Check sheet for the modelled part. Datum: model origin and axes. Units: mm. A direction names the side the tool comes from. Round coordinates to 2 decimals unless told otherwise and drop trailing zeros. Loops run counter-clockwise (first coordinate to the right, second up) from the corner with the lowest first, then second, coordinate; pieces in that order, holes last. Notation, with made-up numbers: (-33, -39.5) - (-12, -39.5) arc R29 ccw to (-12, -7.5) - close; hole circle Ø7 at (10, -29.75). An arc over 180 degrees is marked (long way). Answer in a Markdown table with one row per item. Add a question column.
(1) Cross-section at B-B on z = 0. Enter the section's corners in (x, y), then the cut area to 3 significant figures.
(2) Thickness scan on line 1 along Z through (x, y) = (2.25, 0); line 2 along Z through (x, y) = (-4.25, 4); line 3 along Z through (x, y) = (3.5, 5). Record the ranges inside material, lowest first.
(3) Cross-section at C-C on x = -5. Enter the section's corners in (y, z).
(4) Mould release check, pull along Z, two halves, no side actions. Record for faces 1 (the cylindrical face through (2.46, -0.01, -8.75)), 2 (the flat face through (-8, 2.2, -2.2)), 3 (the cylindrical face through (2.465, 9.895, -0.825)): +Z half, -Z half, draft (parallel to the pull), parting line (faces both ways), or undercut.
(5) Cross-section at A-A on y = 0. Enter the section's corners in (x, z), then the cut area to 3 significant figures.
(6) Access from +Z, -Z, +X, -X, +Y, -Y to the whole of each face (thin tool, end or side, straight path). Record for faces 4 (the cylindrical face through (-3.51, 3.56, -1.62)), 5 (the cylindrical face through (2.465, -7.502, -6.457)), 6 (the cylindrical face through (2.465, -0.825, -9.895)), 7 (the cylindrical face through (2.46, 7.08, 5.14)).
(7) Gauge pin test, flat ends, axial feed: pin 1 (10 mm diameter, centred on y = 3, z = 7, fed in from -X); pin 2 (1.1 mm diameter, centred on x = -6, z = 0, fed in from -Y); pin 3 (3 mm diameter, centred on y = -6.5, z = 6.5, fed in from -X); pin 4 (3 mm diameter, centred on x = -3, z = 0, fed in from +Y). Record the tip position at first contact, or that the pin passes through.
(8) Cross-section at D-D on y = -4. Enter the section's corners in (x, z).
from build123d import *

# Parameters (mm, degrees)
BASPROSKE_W             = 5
BASPROSKE_H             = 11
TOOTHCUT_DEPTH          = 17.340134638
TEETHCUTS_COUNT         = 20
TEETHCUTS_ANGLE         = 342
HUBNEAONESKE_R          = 5
HUBNEARONE_DEPTH        = 10.0000508
BORSKE_R                = 3
BORE_DEPTH              = 15.0000508
BOSS_EXTRUDE1_START     = -10.000051
SKETCH2_R               = 3
BOSS_EXTRUDE1_DEPTH     = 15.0000508
SKETCH3_R               = 1.7
CUT_EXTRUDE1_DEPTH      = 10
SKETCH4_W               = 2
SKETCH4_H               = 20.201666504
CUT_EXTRUDE2_DEPTH      = 19.39087628
CUT_EXTRUDE2_DEPTH_BACK = 19.39087628
CUT_EXTRUDE3_DEPTH      = 31


with BuildPart() as part:
    # BasProSke → Base-Revolve (revolve)
    with BuildSketch(Plane(origin=(0, 0, 0), x_dir=(1, 0, 0), z_dir=(0, 1, 0)), mode=Mode.PRIVATE) as base_revolve_sk:
        with Locations((2.5, 5.5)):
            Rectangle(BASPROSKE_W, BASPROSKE_H)
    revolve(base_revolve_sk.sketch.rotate(Axis((-10, 0, 0), (1, 0, 0)), 180), axis=Axis((-10, 0, 0), (1, 0, 0)))

    # TooCutSke → ToothCut (cut, through all)
    with BuildSketch(Plane(origin=(0, 0, 0), x_dir=(0, 0, -1), z_dir=(1, 0, 0))):
        with BuildLine():
            ThreePointArc((0.589353609, 8.729127295), (0, 8.749), (-0.589353609, 8.729127295))
            ThreePointArc((-0.589353609, 8.729127295), (-0.82475631, 9.893403384), (-1.391689312, 10.937213814))
            ThreePointArc((-1.391689312, 10.937213814), (0, 11.0254), (1.391689312, 10.937213814))
            ThreePointArc((1.391689312, 10.937213814), (0.82475631, 9.893403384), (0.589353609, 8.729127295))
        make_face()
    toothcut = extrude(amount=TOOTHCUT_DEPTH, mode=Mode.SUBTRACT)

    # TeethCuts: ToothCut ×20 about axis
    teethcuts_axis = Axis((-10, 0, 0), (1, 0, 0))
    for i in range(1, TEETHCUTS_COUNT):
        add(toothcut.rotate(teethcuts_axis, i * TEETHCUTS_ANGLE / (TEETHCUTS_COUNT - 1)), mode=Mode.SUBTRACT)

    # HubNeaOneSke → HubNearOne (add)
    with BuildSketch(Plane.ZY):
        with Locations(Location((0, 0, 0), (0, 0, 180))):
            Circle(HUBNEAONESKE_R)
    extrude(amount=HUBNEARONE_DEPTH)

    # BorSke → Bore (cut, symmetric)
    with BuildSketch(Plane(origin=(0, 0, 0), x_dir=(0, 0, -1), z_dir=(1, 0, 0))):
        with Locations(Location((0, 0, 0), (0, 0, 180))):
            Circle(BORSKE_R)
    extrude(amount=BORE_DEPTH, both=True, mode=Mode.SUBTRACT)

    # Sketch2 → Boss-Extrude1 (add)
    with BuildSketch(Plane(origin=(0, 0, 0), x_dir=(0, 0, -1), z_dir=(1, 0, 0)).offset(BOSS_EXTRUDE1_START)):
        Circle(SKETCH2_R)
        with BuildLine():
            Line((-1.65, 2.2), (1.65, 2.2))
            ThreePointArc((1.65, 2.2), (0, -2.75), (-1.65, 2.2))
        make_face(mode=Mode.SUBTRACT)
    extrude(amount=BOSS_EXTRUDE1_DEPTH)

    # Sketch3 → Cut-Extrude1 (cut)
    with BuildSketch(Plane(origin=(0, 0, 0), x_dir=(1, 0, 0), z_dir=(0, 1, 0))):
        with Locations(Location((-3.0000508, 0, 0), (0, 0, 90))):
            Circle(SKETCH3_R)
    extrude(amount=CUT_EXTRUDE1_DEPTH, mode=Mode.SUBTRACT)

    # Sketch4 → Cut-Extrude2 (cut, two sides)
    with BuildSketch(Plane.XY) as cut_extrude2_sk:
        with Locations((-9.0000508, 0)):
            Rectangle(SKETCH4_W, SKETCH4_H)
    extrude(amount=CUT_EXTRUDE2_DEPTH, mode=Mode.SUBTRACT)
    extrude(cut_extrude2_sk.sketch, amount=-CUT_EXTRUDE2_DEPTH_BACK, mode=Mode.SUBTRACT)

    # Sketch5 → Cut-Extrude3 (cut)
    with BuildSketch(Plane.ZY.offset(8.0000508)):
        with BuildLine():
            Line((1.145643924, 2.5), (0, 2.5))
            Line((0, 2.5), (-1.145643924, 2.5))
            ThreePointArc((-1.145643924, 2.5), (-1.40584716, 2.363491858), (-1.65, 2.2))
            Line((-1.65, 2.2), (1.65, 2.2))
            ThreePointArc((1.65, 2.2), (1.40584716, 2.363491858), (1.145643924, 2.5))
        make_face()
    extrude(amount=-CUT_EXTRUDE3_DEPTH, mode=Mode.SUBTRACT)


solid = part.part
Answers:
| question | item | result |
|---|---|---|
| 1 | outline | (-8, -5) - (0, -5) - (0, -8.75) - (5, -8.75) - (5, -2.75) - (-8, -2.75) - close; (-8, 2.5) - (-4.7, 2.5) - (-4.7, 5) - (-8, 5) - close; (-1.3, 2.5) - (5, 2.5) - (5, 8.75) - (0, 8.75) - (0, 5) - (-1.3, 5) - close |
| 1 | area | 90.7 mm^2 |
| 2 | line 1 | z = -8.75 to -2.75, 2.75 to 8.75 |
| 2 | line 2 | z = -3 to -1.15, 1.15 to 3 |
| 2 | line 3 | z = -9.8 to -8.06, -7.18 to 7.18, 8.06 to 9.8 |
| 3 | outline | circle Ø10 at (0, 0); hole (2.5, -1.15) - (2.5, 1.15) arc R2.75 ccw (long way) to start |
| 4 | face 1 | -Z half |
| 4 | face 2 | draft |
| 4 | face 3 | undercut |
| 5 | outline | (-8, -5) - (0, -5) - (0, -8.75) - (5, -8.75) - (5, -2.75) - (-8, -2.75) - close; (-8, 2.75) - (5, 2.75) - (5, 8.75) - (0, 8.75) - (0, 5) - (-8, 5) - close |
| 5 | area | 96.0 mm^2 |
| 6 | face 4 | +Y |
| 6 | face 5 | +X, -X, -Y |
| 6 | face 6 | -Z, +X, -X |
| 6 | face 7 | +X, -X |
| 7 | pin 1 | stops at x = -8 |
| 7 | pin 2 | stops at y = -5 |
| 7 | pin 3 | stops at x = 0 |
| 7 | pin 4 | stops at y = -2.3 |
| 8 | outline | (-8, -3) - (0, -3) - (0, -9.34) - (5, -9.34) - (5, 9.34) - (0, 9.34) - (0, 3) - (-8, 3) - close |
